Model file for the job. Use its own axes, mm. Face numbers are marked on the shaded views. Round coordinates to 2 decimals unless told otherwise and drop trailing zeros. Order: outer loops, then holes, each group sorted by start corner. A loop starts at its lowest first (then second) coordinate and runs counter-clockwise, first axis right, second up. Notation, with made-up numbers: (-3.75, 60) - (28.25, 60) arc R36 cw to (28.25, 99) - close; hole circle Ø6 at (82.25, 38). An arc over 180 degrees is marked (long way). Put each result on its own line as item: value. Start each with the question number.
Item 1: Mould opens along Z. For the marked faces 1 and 2 say: pulls with the +Z half, pulls with the -Z half, needs draft (parallel to the pull), parting line crosses it, or undercut.
Item 2: Saw through at B-B on x = 0. List the corners of the cut face in (y, z) (3 decimals), plus the area to 3 significant figures.
Item 3: Saw through at D-D on y = 13.5. List the corners of the cut face in (x, z) (3 decimals).
Item 4: Pin check, flat tips, straight feed: pin 1 Ø1.5 at (x, y) = (8, 23.5) entering from +Z; pin 2 Ø1.5 at (x, y) = (-9.5, 100) entering from -Z; pin 3 Ø2 at (y, z) = (13.5, -13) entering from +X (3 decimals). Stop position of each tip, or through.
Item 5: Saw through at C-C on y = 79. List the corners of the cut face in (x, z) (3 decimals).
Item 6: Probe probe 1 along Z at (x, y) = (0, 56.5) (3 decimals); probe 2 along X at (y, z) = (57, -0.25); probe 3 along X at (y, z) = (81, 9). List the from-to ranges inside material, lowest first.
Item 7: Saw through at A-A on z = 0. List the corners of the cut face in (x, y) (3 decimals).
```python
from build123d import *

# Parameters (mm, degrees)
SKETCH1_R           = 14.605
SKETCH1_R_2         = 12.065
BOSS_EXTRUDE1_DEPTH = 146.05
SKETCH2_W           = 3.556
SKETCH2_H           = 25.4
CUT_EXTRUDE1_DEPTH  = 25.4


with BuildPart() as part:
    # Sketch1 → Boss-Extrude1 (new body)
    with BuildSketch(Plane(origin=(0, 0, 0), x_dir=(1, 0, 0), z_dir=(0, 1, 0))):
        with Locations(Location((0, 0, 0), (0, 0, 270))):
            Circle(SKETCH1_R)
        with Locations(Location((0, 0, 0), (0, 0, 270))):
            Circle(SKETCH1_R_2, mode=Mode.SUBTRACT)
    extrude(amount=BOSS_EXTRUDE1_DEPTH)

    # Sketch2 → Cut-Extrude1 (cut)
    with BuildSketch(Plane.XY):
        with Locations((0, 12.7)):
            Rectangle(SKETCH2_W, SKETCH2_H)
    extrude(amount=-CUT_EXTRUDE1_DEPTH, mode=Mode.SUBTRACT)


solid = part.part
```
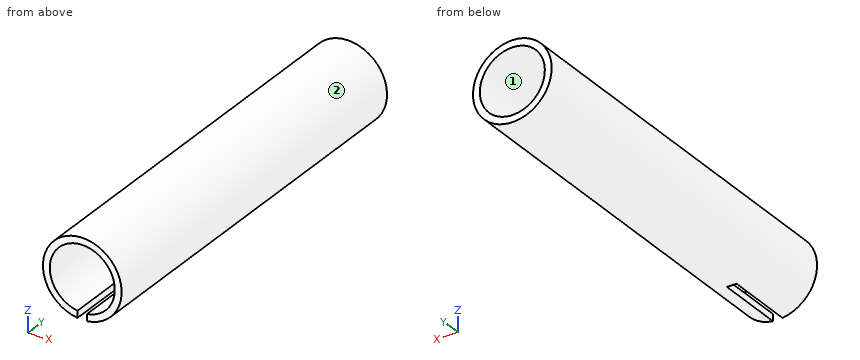
Results found:
1. face 1: undercut
1. face 2: parting line crosses it
2. outline: (0, 12.065) - (146.05, 12.065) - (146.05, 14.605) - (0, 14.605) - close; (25.4, -14.605) - (146.05, -14.605) - (146.05, -12.065) - (25.4, -12.065) - close
2. area: 677 mm²
3. outline: (-1.778, -14.496) - (-1.778, -11.933) arc R12.065 cw (long way) to (1.778, -11.933) - (1.778, -14.496) arc R14.605 ccw (long way) to start
4. pin 1: stops at z = 12.68
4. pin 2: stops at z = -11.69
4. pin 3: stops at x = 8.325
5. outline: circle Ø29.21 at (0, 0); hole circle Ø24.13 at (0, 0)
6. probe 1: z = -14.605 to -12.065, 12.065 to 14.605
6. probe 2: x = -14.6 to -12.06, 12.06 to 14.6
6. probe 3: x = -11.5 to -8.04, 8.04 to 11.5
7. outline: (-14.605, 0) - (-12.065, 0) - (-12.065, 146.05) - (-14.605, 146.05) - close; (12.065, 0) - (14.605, 0) - (14.605, 146.05) - (12.065, 146.05) - close
